```python
from build123d import *

# Parameters (mm, degrees)
CROQUIS1_W              = 86
CROQUIS1_H              = 30
SALIENTE_EXTRUIR1_DEPTH = 3
CORTAR_EXTRUIR1_REACH   = 5
CROQUIS2_R              = 2
CROQUIS2_W              = 3
CROQUIS2_H              = 10
REDONDEO1_R             = 10


with BuildPart() as part:
    # Croquis1 → Saliente-Extruir1 (new body)
    with BuildSketch(Plane.XY):
        Rectangle(CROQUIS1_W, CROQUIS1_H)
    extrude(amount=SALIENTE_EXTRUIR1_DEPTH)

    # Croquis2 → Cortar-Extruir1 (cut, up to next)
    with BuildSketch(Plane.XY.offset(3), mode=Mode.PRIVATE) as cortar_extruir1_sk1:
        with Locations((-19, 6)):
            Circle(CROQUIS2_R)
    cortar_extruir1_tool1 = extrude(cortar_extruir1_sk1.sketch, amount=-CORTAR_EXTRUIR1_REACH, mode=Mode.PRIVATE) & part.part
    add(cortar_extruir1_tool1.solids().sort_by_distance((-19, 6, 3))[0], mode=Mode.SUBTRACT)
    # Croquis2 → Cortar-Extruir1 (cut, up to next)
    with BuildSketch(Plane.XY.offset(3), mode=Mode.PRIVATE) as cortar_extruir1_sk2:
        with Locations((-19, -6)):
            Circle(CROQUIS2_R)
    cortar_extruir1_tool2 = extrude(cortar_extruir1_sk2.sketch, amount=-CORTAR_EXTRUIR1_REACH, mode=Mode.PRIVATE) & part.part
    add(cortar_extruir1_tool2.solids().sort_by_distance((-19, -6, 3))[0], mode=Mode.SUBTRACT)
    # Croquis2 → Cortar-Extruir1 (cut, up to next)
    with BuildSketch(Plane.XY.offset(3), mode=Mode.PRIVATE) as cortar_extruir1_sk3:
        with Locations((-31, 0)):
            Rectangle(CROQUIS2_W, CROQUIS2_H)
    cortar_extruir1_tool3 = extrude(cortar_extruir1_sk3.sketch, amount=-CORTAR_EXTRUIR1_REACH, mode=Mode.PRIVATE) & part.part
    add(cortar_extruir1_tool3.solids().sort_by_distance((-31, 0, 3))[0], mode=Mode.SUBTRACT)
    # Croquis2 → Cortar-Extruir1 (cut, up to next)
    with BuildSketch(Plane.XY.offset(3), mode=Mode.PRIVATE) as cortar_extruir1_sk4:
        with Locations((31, 0)):
            Rectangle(CROQUIS2_W, CROQUIS2_H)
    cortar_extruir1_tool4 = extrude(cortar_extruir1_sk4.sketch, amount=-CORTAR_EXTRUIR1_REACH, mode=Mode.PRIVATE) & part.part
    add(cortar_extruir1_tool4.solids().sort_by_distance((31, 0, 3))[0], mode=Mode.SUBTRACT)

    # Redondeo1
    redondeo1_edges = [part.edges().sort_by_distance(p)[0] for p in [
        (43, -15, 1.5),
        (-43, -15, 1.5),
        (-43, 15, 1.5),
        (43, 15, 1.5),
    ]]
    fillet(redondeo1_edges, radius=REDONDEO1_R)


solid = part.part
```
The listing builds one solid part. Answer for the finished solid, in the listing's coordinates (mm). A direction names the side the tool comes from. Coordinates: 2 decimals unless noted, no trailing zeros. Loops run counter-clockwise (first coordinate to the right, second up) from the corner with the lowest first, then second, coordinate; pieces in that order, holes last. Notation, with made-up numbers: (-26.5, 37) - (26.5, 37) arc R29 ccw to (26.5, 70) - close; hole circle Ø8 at (78.25, -20). An arc over 180 degrees is marked (long way). Use a Markdown table: item, result. Add a question column.
1) The part is cut by section D-D, the plane y = -11. Give the vertices of the cut face in (x, z), and give its area (3 significant figures).
2) For faces 4 (the flat face through (31, 5, 2)), 5 (the cylindrical face through (39.99, 12.15, 1.52)), determine the directions among +Z, -Z, +X, -X, +Y, -Y from which every point of the face is accessible in a straight line to the end or side of a thin tool.
3) Find the intervals of material crossed by line 1 (Y direction, x = -19, z = 1.45); line 2 (X direction, y = 2.5, z = 0.4); line 3 (X direction, y = 7.5, z = 2.85), in increasing order.
4) Given pin 1 (3.5 mm diameter, centred on x = -19, y = 6, fed in from +Z); pin 2 (1 mm diameter, centred on y = 12, z = 2.5, fed in from -X), each flat-ended and moving along its own axis, determine where each tip first touches the part or whether it passes through.
5) The part is cut by section B-B, the plane z = 1. Give the vertices of the cut face in (x, y).
6) The mould has two halves that part along X. Classify faces 1 (the flat face through (32.5, 0, 2)), 2 (the flat face through (-1, 0, 3)), 3 (the cylindrical face through (39.99, -12.15, 1.52)): released by +X, released by -X, zero draft, split by the parting line, or undercut.
7) The part is cut by section A-A, the plane x = -19. Give the vertices of the cut face in (y, z).
8) The part is cut by section C-C, the plane y = 6. Give the vertices of the cut face in (x, z), and give its area (3 significant figures).
Here are the results:
| question | item | result |
|---|---|---|
| 1 | outline | (-41, 0) - (41, 0) - (41, 3) - (-41, 3) - close |
| 1 | area | 246 mm^2 |
| 2 | face 4 | +Z, -Z |
| 2 | face 5 | +Z, -Z, +X, +Y |
| 3 | line 1 | y = -15 to -8, -4 to 4, 8 to 15 |
| 3 | line 2 | x = -43 to -32.5, -29.5 to 29.5, 32.5 to 43 |
| 3 | line 3 | x = -42.68 to -20.32, -17.68 to 42.68 |
| 4 | pin 1 | passes through |
| 4 | pin 2 | stops at x = -40.6 |
| 5 | outline | (-43, -5) arc R10 ccw to (-33, -15) - (33, -15) arc R10 ccw to (43, -5) - (43, 5) arc R10 ccw to (33, 15) - (-33, 15) arc R10 ccw to (-43, 5) - close; hole (-32.5, -5) - (-29.5, -5) - (-29.5, 5) - (-32.5, 5) - close; hole circle Ø4 at (-19, -6); hole circle Ø4 at (-19, 6); hole (29.5, -5) - (32.5, -5) - (32.5, 5) - (29.5, 5) - close |
| 6 | face 1 | undercut |
| 6 | face 2 | zero draft |
| 6 | face 3 | released by +X |
| 7 | outline | (-15, 0) - (-8, 0) - (-8, 3) - (-15, 3) - close; (-4, 0) - (4, 0) - (4, 3) - (-4, 3) - close; (8, 0) - (15, 0) - (15, 3) - (8, 3) - close |
| 8 | outline | (-42.95, 0) - (-21, 0) - (-21, 3) - (-42.95, 3) - close; (-17, 0) - (42.95, 0) - (42.95, 3) - (-17, 3) - close |
| 8 | area | 246 mm^2 |
